from build123d import *

# Parameters (mm, degrees)
F1_DEPTH  = 5.4
F2_R      = 5.05
F2_R_2    = 3.05
F3_DEPTH  = 0.4
F4_R      = 2
F5_DEPTH  = 5.401
F6_R      = 3.5
F6_R_2    = 2
F7_DEPTH  = 0.5
F8_R      = 2.5
F9_DEPTH  = 4.5
F11_DEPTH = 5


with BuildPart() as f1:
    # F0 (on Top) → F1 (new body)
    with BuildSketch(Plane.XY):
        Polygon((6, -3.4641016151), (6, 3.4641016151), (0, 6.9282032303), (-6, 3.4641016151), (-6, -3.4641016151), (0, -6.9282032303), align=None)
    extrude(amount=F1_DEPTH)

    # F2 (on face) → F3 (cut)
    with BuildSketch(Plane.XY.offset(5.4)):
        Circle(F2_R)
        Circle(F2_R_2, mode=Mode.SUBTRACT)
    extrude(amount=-F3_DEPTH, mode=Mode.SUBTRACT)

    # F4 (on face) → F5 (cut, through all)
    with BuildSketch(Plane.XY.offset(5.4)):
        Circle(F4_R)
    extrude(amount=-F5_DEPTH, mode=Mode.SUBTRACT)

    # F6 (on face) → F7 (join)
    with BuildSketch(Plane(origin=(0, 0, 0), x_dir=(1, 0, 0), z_dir=(0, 0, -1))):
        Circle(F6_R)
        Circle(F6_R_2, mode=Mode.SUBTRACT)
    extrude(amount=F7_DEPTH)

    # F8 (on face) → F9 (cut)
    with BuildSketch(Plane(origin=(0, 0, -0.5), x_dir=(1, 0, 0), z_dir=(0, 0, -1))):
        Circle(F8_R)
    extrude(amount=-F9_DEPTH, mode=Mode.SUBTRACT)

    # F10 (on Right) → F11 (cut, symmetric)
    with BuildSketch(Plane.YZ):
        with BuildLine():
            Line((1, -1.5), (1, 1.2))
            ThreePointArc((1, 1.2), (0, 2.2), (-1, 1.2))
            Line((-1, 1.2), (-1, -1.5))
            Line((-1, -1.5), (1, -1.5))
        make_face()
    extrude(amount=F11_DEPTH, both=True, mode=Mode.SUBTRACT)


solid = f1.part
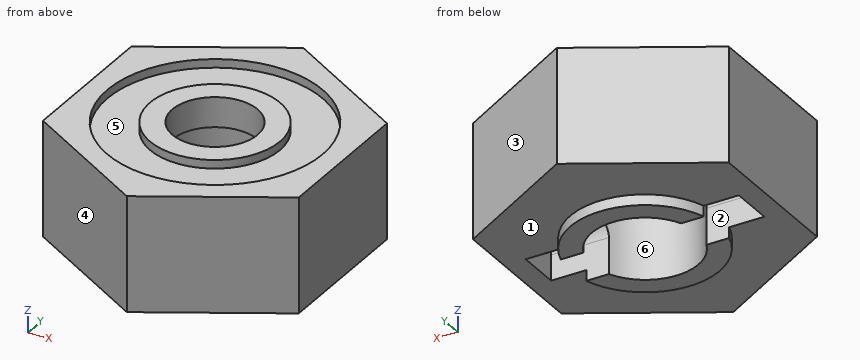
The model under review builds one solid part; all positions refer to its coordinate system, in mm. Face numbers are marked on the shaded views. A direction names the side the tool comes from. Give positions to 0.01 mm unless a question says otherwise; leave off trailing zeros. Order: outer loops, then holes, each group sorted by start corner. A loop starts at its lowest first (then second) coordinate and runs counter-clockwise, first axis right, second up. Notation, with made-up numbers: M 62.25,83.5 L 76.25,83.5 A18 ccw 76.25,105.5 Z; hole C 8.25,-25.5 d1. An arc over 180 degrees is marked long. One line per question, with ' | ' between items. Start each with the question number.
1) Consider section B-B, the plane x = 1. Give the boundary of the cut face in (y, z), then the cut area to 3 significant figures.
2) For the marked faces 4, 5 and 6, list the 3-axis set-ups (+Z, -Z, +X, -X, +Y, -Y) from which the entire face can be reached by the end or side of a thin tool; tool diameter is ignored.
3) Consider section A-A, the plane y = 0. Give the boundary of the cut face in (x, z), then the cut area to 3 significant figures.
4) Wall thickness on L1, parallel to X at y = -0.5, z = 1.05; L2, parallel to X at y = 0, z = 2.9; L3, parallel to Z at x = 0.75, y = 4: over which ranges is each line inside the solid? List them lowest first. Write a range as from..to.
5) Mouldability with a two-part tool opening along Y and no side actions: class the marked faces 1, 2 and 3 as pulls with the +Y half, pulls with the -Y half, needs draft (parallel to the pull), parting line crosses it, or undercut.
6) Consider section C-C, the plane z = 4.45. Give the boundary of the cut face in (x, y).
7) Consider section D-D, the plane y = -4. Give the boundary of the cut face in (x, z), then the cut area to 3 significant figures.
8) Clearance check with flat-ended pins moving along their axes: P1, Ø1.4, axis at x = 4, z = 0.5, coming from the -Y side; P2, Ø0.8, axis at x = 3.5, z = 0, coming from the +Y side; P3, Ø1.4, axis at x = -3, z = 1, coming from the +Y side. State where each tip first meets the part, or that it passes through.
Found:
1) outline: M -6.35,0 L -3.35,0 L -3.35,-0.5 L -2.29,-0.5 L -2.29,4 L -1.73,4 L -1.73,5.4 L -2.88,5.4 L -2.88,5 L -4.95,5 L -4.95,5.4 L -6.35,5.4 Z; M 1.73,4 L 2.29,4 L 2.29,-0.5 L 3.35,-0.5 L 3.35,0 L 6.35,0 L 6.35,5.4 L 4.95,5.4 L 4.95,5 L 2.88,5 L 2.88,5.4 L 1.73,5.4 Z | area: 44.8 mm²
2) face 4: +Z, -Z, -X, -Y | face 5: +Z | face 6: -Z
3) outline: M -6,0 L -5,0 L -5,2.2 L -2.5,2.2 L -2.5,4 L -2,4 L -2,5.4 L -3.05,5.4 L -3.05,5 L -5.05,5 L -5.05,5.4 L -6,5.4 Z; M 2,4 L 2.5,4 L 2.5,2.2 L 5,2.2 L 5,0 L 6,0 L 6,5.4 L 5.05,5.4 L 5.05,5 L 3.05,5 L 3.05,5.4 L 2,5.4 Z | area: 26.6 mm²
4) L1: x = -6..-5, 5..6 | L2: x = -6..-2.5, 2.5..6 | L3: z = 0..5
5) face 1: needs draft | face 2: undercut | face 3: pulls with the +Y half
6) outline: M -6,-3.46 L 0,-6.93 L 6,-3.46 L 6,3.46 L 0,6.93 L -6,3.46 Z; hole C 0,0 d4
7) outline: M -5.07,0 L 5.07,0 L 5.07,5.4 L 3.08,5.4 L 3.08,5 L -3.08,5 L -3.08,5.4 L -5.07,5.4 Z | area: 52.3 mm²
8) P1: stops at y = -5.02 | P2: stops at y = 5.14 | P3: stops at y = 5.6
